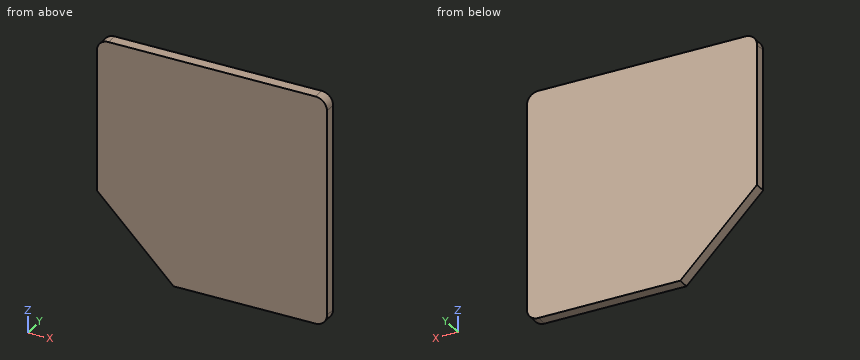
```python
from build123d import *

# Parameters (mm, degrees)
F1_DEPTH = 6
F2_R     = 6
F3_R     = 6


with BuildPart() as f1:
    # F0 (on Front) → F1 (new body)
    with BuildSketch(Plane.XZ):
        Polygon((0, -120), (0, 0), (-120, 0), (-120, -80), (-80, -120), align=None)
    extrude(amount=F1_DEPTH)

    # F2
    f2_edges = [f1.edges().sort_by_distance(p)[0] for p in [
        (0, -3, 0),
    ]]
    fillet(f2_edges, radius=F2_R)

    # F3
    f3_edges = [f1.edges().sort_by_distance(p)[0] for p in [
        (-120, -3, 0),
        (0, -3, -120),
    ]]
    fillet(f3_edges, radius=F3_R)


solid = f1.part
```
Part model, mm, in its own coordinate system. Round coordinates to 2 decimals unless told otherwise and drop trailing zeros. Loops run counter-clockwise (first coordinate to the right, second up) from the corner with the lowest first, then second, coordinate; pieces in that order, holes last.
Item 1: Drill centre lines: line 1 (X direction, y = -2.2, z = -108); line 2 (X direction, y = -4.95, z = -103.5); line 3 (Z direction, x = -101, y = -1.3). Where is each one in solid material? Low to high.
Item 2: Cut at B-B, the plane x = -112. Give the cut face in (y, z), then the cut area to 3 significant figures.
Item 3: Cut at A-A, the plane y = -3.8. Give the cut face in (x, z), then the cut area to 3 significant figures.
Item 4: Cut at C-C, the plane x = -97. Give the cut face in (y, z), then the cut area to 3 significant figures.
A:
1. line 1: x = -92 to 0
1. line 2: x = -96.5 to 0
1. line 3: z = -99 to 0
2. outline: (-6, -88) - (0, -88) - (0, 0) - (-6, 0) - close
2. area: 528 mm2
3. outline: (-120, -80) - (-80, -120) - (-6, -120) arc R6 ccw to (0, -114) - (0, -6) arc R6 ccw to (-6, 0) - (-114, 0) arc R6 ccw to (-120, -6) - close
3. area: 13,600 mm2
4. outline: (-6, -103) - (0, -103) - (0, 0) - (-6, 0) - close
4. area: 618 mm2
